The model under review builds one solid part; all positions refer to its coordinate system, in mm. Face numbers are marked on the shaded views. A direction names the side the tool comes from. Coordinates: 2 decimals unless noted, no trailing zeros. Order: outer loops, then holes, each group sorted by start corner. A loop starts at its lowest first (then second) coordinate and runs counter-clockwise, first axis right, second up. Notation, with made-up numbers: (-20.75, 62.5) -> (-1.75, 62.5) arc R17 ccw to (-1.75, 73.5) -> close; hole circle Ø2 at (58.25, 61.25). An arc over 180 degrees is marked (long way). Use one line per item in the form item = value. Start each with the question number.
(1) Mouldability with a two-part tool opening along Y and no side actions: class the marked faces 4, 5, 6 and 7 as +Y half, -Y half, draft (parallel to the pull), parting line (faces both ways), or undercut.
(2) Insertion check: pin 1 Ø8 at (y, z) = (41.5, -39) entering from +X (3 decimals); pin 2 Ø3.5 at (x, y) = (79.5, 17) entering from +Z; pin 3 Ø9.5 at (x, z) = (4.5, -9.5) entering from +Y; pin 4 Ø6 at (x, y) = (78, 10.5) entering from -Z. Each pin has a flat end and moves straight along its axis. Give the tip position at first contact, or say it passes through.
(3) Take a section at B-B (z = -15.5). State the section outline as (x, y) points.
(4) Wall thickness on line 1 along X through (y, z) = (1.15, -24); line 2 along Y through (x, z) = (75.5, -35.5); line 3 along Y through (x, z) = (79.5, -11): over which ranges is each line inside the solid? List them lowest first.
(5) Take a section at C-C (z = -6). State the section outline as (x, y) points.
(6) Take a section at A-A (x = 79.5). State the section outline as (y, z) points, then the cut area to 3 significant figures.
(7) For the marked faces 1, 2 and 3, list the 3-axis set-ups (+Z, -Z, +X, -X, +Y, -Y) from which the entire face can be reached by the end or side of a thin tool; tool diameter is ignored.
(8) Take a section at D-D (y = 43). State the section outline as (x, z) points.
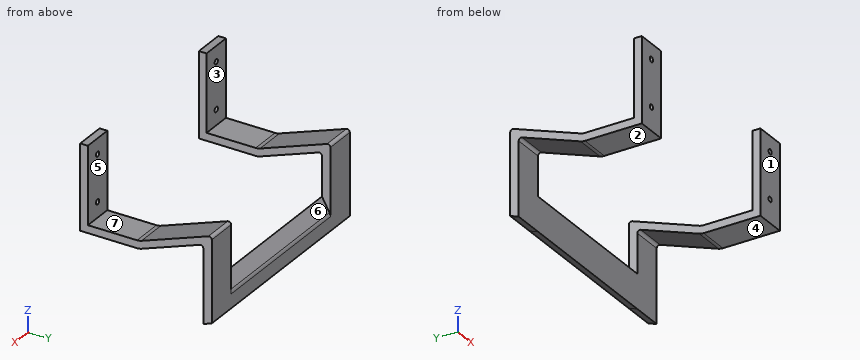
```python
from build123d import *

# Parameters (mm, degrees)
SKETCH1_W             = 12
SKETCH1_H             = 33
SKETCH1_R             = 1
BOSS_EXTRUDE1_DEPTH   = 3
BOSS_EXTRUDE1_2_DEPTH = 3
SKETCH2_W             = 12
SKETCH2_H             = 3
BOSS_EXTRUDE2_DEPTH   = 20
SKETCH3_W             = 12
SKETCH3_H             = 3
BOSS_EXTRUDE3_DEPTH   = 30
SKETCH5_W             = 12
SKETCH5_H             = 3.5
BOSS_EXTRUDE4_DEPTH   = 30
BOSS_EXTRUDE5_DEPTH   = 61.5
FILLET2_R             = 1
FILLET3_R             = 3
FILLET4_R             = 5
FILLET5_R             = 5
FILLET6_R             = 1


with BuildPart() as part:
    # Sketch1 → Boss-Extrude1 (new body)
    with BuildSketch(Plane(origin=(0, 0, 0), x_dir=(1, 0, 0), z_dir=(0, 1, 0))):
        with Locations((6, 16.5)):
            Rectangle(SKETCH1_W, SKETCH1_H)
        with Locations((6, 24)):
            Circle(SKETCH1_R, mode=Mode.SUBTRACT)
        with Locations((6, 6)):
            Circle(SKETCH1_R, mode=Mode.SUBTRACT)
    extrude(amount=BOSS_EXTRUDE1_DEPTH)



with BuildPart() as body_2:
    # Sketch1 → Boss-Extrude1 2 (new body)
    with BuildSketch(Plane(origin=(0, 0, 0), x_dir=(1, 0, 0), z_dir=(0, 1, 0))):
        with Locations((79.5, 16.5)):
            Rectangle(SKETCH1_W, SKETCH1_H)
        with Locations((79.5, 24)):
            Circle(SKETCH1_R, mode=Mode.SUBTRACT)
        with Locations((79.5, 6)):
            Circle(SKETCH1_R, mode=Mode.SUBTRACT)
    extrude(amount=BOSS_EXTRUDE1_2_DEPTH)


with BuildPart() as part_1:
    add(part.part)

    add(body_2.part)  # Boss-Extrude2 merges body 2
    # Sketch2 → Boss-Extrude2 (add)
    with BuildSketch(Plane(origin=(0, 3, 0), x_dir=(1, 0, 0), z_dir=(0, 1, 0))):
        with Locations((6, 31.5)):
            Rectangle(SKETCH2_W, SKETCH2_H)
        with Locations((79.5, 31.5)):
            Rectangle(SKETCH2_W, SKETCH2_H)
    extrude(amount=BOSS_EXTRUDE2_DEPTH)

    # Sketch3 → Boss-Extrude3 (add, along a direction that is not the sketch's normal)
    with BuildSketch(Plane(origin=(0, 23, 0), x_dir=(1, 0, 0), z_dir=(0, 1, 0))):
        with Locations((79.5, 31.5)):
            Rectangle(SKETCH3_W, SKETCH3_H)
        with Locations((6, 31.5)):
            Rectangle(SKETCH3_W, SKETCH3_H)
    extrude(amount=BOSS_EXTRUDE3_DEPTH, dir=(0, 0.939692621, 0.342020143))

    # Sketch5 → Boss-Extrude4 (add, along a direction that is not the sketch's normal)
    with BuildSketch(Plane(origin=(0, 13.296484464, -36.531790823), x_dir=(-1, 0, 0), z_dir=(0, 0.342020143, -0.939692621))):
        with Locations((-79.5, 38.576265548)):
            Rectangle(SKETCH5_W, SKETCH5_H)
        with Locations((-6, 38.576265548)):
            Rectangle(SKETCH5_W, SKETCH5_H)
    extrude(amount=BOSS_EXTRUDE4_DEPTH, dir=(0, 0, -1))

    # Sketch6 → Boss-Extrude5 (add)
    with BuildSketch(Plane(origin=(12, 0, 0), x_dir=(0, 0, -1), z_dir=(1, 0, 0))):
        Polygon((53.936466202, 47.901854451), (52.7393957, 51.190778624), (46.533858727, 51.190778624), (40.660160277, 47.901854451), align=None)
    extrude(amount=BOSS_EXTRUDE5_DEPTH)

    # Fillet2
    fillet2_edges = [part_1.edges().sort_by_distance(p)[0] for p in [
        (6, 51.190778624, -19.7393957),
        (79.5, 51.190778624, -19.7393957),
    ]]
    fillet(fillet2_edges, radius=FILLET2_R)

    # Fillet3
    fillet3_edges = [part_1.edges().sort_by_distance(p)[0] for p in [
        (42.75, 51.190778624, -46.533858727),
    ]]
    fillet(fillet3_edges, radius=FILLET3_R)

    # Fillet4
    fillet4_edges = [part_1.edges().sort_by_distance(p)[0] for p in [
        (6, 23, -33),
        (79.5, 23, -33),
    ]]
    fillet(fillet4_edges, radius=FILLET4_R)

    # Fillet5
    fillet5_edges = [part_1.edges().sort_by_distance(p)[0] for p in [
        (6, 23, -30),
        (79.5, 23, -30),
    ]]
    fillet(fillet5_edges, radius=FILLET5_R)

    # Fillet6
    fillet6_edges = [part_1.edges().sort_by_distance(p)[0] for p in [
        (6, 47.901854451, -23.936466202),
        (79.5, 47.901854451, -23.936466202),
    ]]
    fillet(fillet6_edges, radius=FILLET6_R)


solid = part_1.part
```
Findings:
q1.face_4 = draft
q1.face_5 = undercut
q1.face_6 = +Y half
q1.face_7 = undercut
q2.pin_1 = through
q2.pin_2 = -30
q2.pin_3 = 3
q2.pin_4 = -33
q3.outline = (0, 0) -> (12, 0) -> (12, 3) -> (0, 3) -> close; (73.5, 0) -> (85.5, 0) -> (85.5, 3) -> (73.5, 3) -> close
q4.line_1 = 0 to 5, 7 to 12, 73.5 to 78.5, 80.5 to 85.5
q4.line_2 = 47.9 to 51.19
q4.line_3 = 0 to 3
q5.outline = (0, 0) -> (5, 0) -> (5, 3) -> (0, 3) -> close; (7, 0) -> (12, 0) -> (12, 3) -> (7, 3) -> close; (73.5, 0) -> (78.5, 0) -> (78.5, 3) -> (73.5, 3) -> close; (80.5, 0) -> (85.5, 0) -> (85.5, 3) -> (80.5, 3) -> close
q6.outline = (0, -33) -> (22.12, -33) arc R5 ccw to (23.83, -32.7) -> (46.56, -24.42) arc R1 cw to (47.9, -25.36) -> (47.9, -53.94) -> (51.19, -52.74) -> (51.19, -21.17) arc R1 ccw to (49.85, -20.23) -> (23.83, -29.7) arc R5 cw to (22.12, -30) -> (3, -30) -> (3, -25) -> (0, -25) -> close; (0, -23) -> (3, -23) -> (3, -7) -> (0, -7) -> close; (0, -5) -> (3, -5) -> (3, 0) -> (0, 0) -> close
q6.area = 330 mm²
q7.face_1 = +Z, -Z, +X, -X, -Y
q7.face_2 = -Z, +X, -X, -Y
q7.face_3 = +Z, +X, -X
q8.outline = (0, -25.72) -> (12, -25.72) -> (12, -22.72) -> (0, -22.72) -> close; (73.5, -25.72) -> (85.5, -25.72) -> (85.5, -22.72) -> (73.5, -22.72) -> close
